Design review of the part built by this model. Coordinates are the model's own, in mm. Give positions to 0.01 mm unless a question says otherwise; leave off trailing zeros. Loops run counter-clockwise (first coordinate to the right, second up) from the corner with the lowest first, then second, coordinate; pieces in that order, holes last. Notation, with made-up numbers: M 31,-6.5 L 59,-6.5 A24 cw 59,31.5 Z; hole C -32.5,85.25 d4. An arc over 180 degrees is marked long. Use CSV: the item, a comma, the result in double quotes.
from build123d import *

# Parameters (mm, degrees)
SKETCH1_R           = 2.4892
SKETCH1_R_2         = 2.5527
BOSS_EXTRUDE1_DEPTH = 3.175
SKETCH2_W           = 4.445
SKETCH2_H           = 39.37
CUT_EXTRUDE1_DEPTH  = 4.175
FILLET2_R           = 4.7625


with BuildPart() as part:
    # Sketch1 → Boss-Extrude1 (new body)
    with BuildSketch(Plane.XY):
        Polygon((-34.925, 31.75), (-34.925, -29.21), (34.925, -29.21), (34.925, -7.62), (-10.795, -7.62), (-10.795, 31.75), align=None)
        with Locations((-25.4, -19.05)):
            Circle(SKETCH1_R, mode=Mode.SUBTRACT)
        with Locations((-7.874, -19.05)):
            Circle(SKETCH1_R, mode=Mode.SUBTRACT)
        with Locations((-25.4, -6.35)):
            Circle(SKETCH1_R, mode=Mode.SUBTRACT)
        with Locations((4.826, -19.05)):
            Circle(SKETCH1_R_2, mode=Mode.SUBTRACT)
        with Locations((17.526, -19.05)):
            Circle(SKETCH1_R_2, mode=Mode.SUBTRACT)
        with Locations((-25.4, 6.35)):
            Circle(SKETCH1_R, mode=Mode.SUBTRACT)
        with Locations((-25.4, 19.05)):
            Circle(SKETCH1_R, mode=Mode.SUBTRACT)
        with Locations((-25.4, -19.05)):
            Circle(SKETCH1_R)
    extrude(amount=BOSS_EXTRUDE1_DEPTH)

    # Sketch2 → Cut-Extrude1 (cut, through all)
    with BuildSketch(Plane.XY.offset(3.175)):
        with Locations((-13.0175, 12.065)):
            Rectangle(SKETCH2_W, SKETCH2_H)
    extrude(amount=-CUT_EXTRUDE1_DEPTH, mode=Mode.SUBTRACT)

    # Fillet2
    fillet2_edges = [part.edges().sort_by_distance(p)[0] for p in [
        (-34.925, 31.75, 1.5875),
        (34.925, -7.62, 1.5875),
        (34.925, -29.21, 1.5875),
        (-34.925, -29.21, 1.5875),
        (-15.24, -7.62, 1.5875),
        (-15.24, 31.75, 1.5875),
    ]]
    fillet(fillet2_edges, radius=FILLET2_R)


solid = part.part
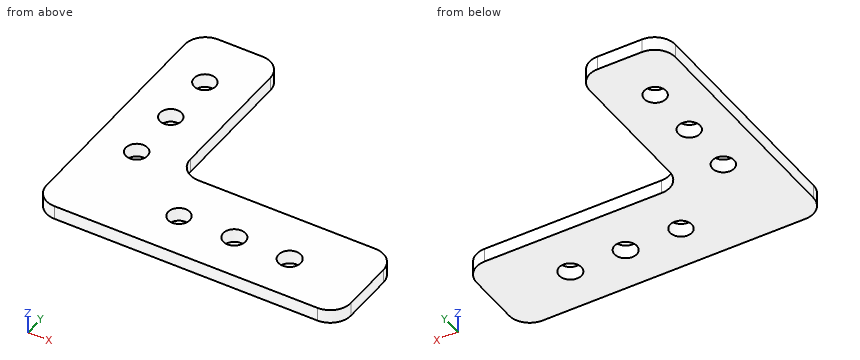
(1) We need section B-B on y = 19.05. State the section outline as (x, z) points (3 decimals), then the cut area to 3 significant figures.
A:
outline,"M -34.925,0 L -27.889,0 L -27.889,3.175 L -34.925,3.175 Z; M -22.911,0 L -15.24,0 L -15.24,3.175 L -22.911,3.175 Z"
area,"46.7 mm²"
(2) We need section C-C on z = 0.6. Count the separate pieces of the cut face and the enclosed holes in it, then the cut area to 3 significant figures.
A:
separate pieces,"1"
enclosed holes,"6"
area,"2,140 mm²"
(3) Clearance check with a flat-ended pin moving along its axis: P1, Ø6.5, axis at x = -25.4, y = 19.05, coming from the +Z side (3 decimals). State where the tip first meets the part, or that it passes through.
A:
P1,"z = 3.175"
(4) We need section D-D on x = 10.5. State the section outline as (y, z) points (3 decimals).
A:
outline,"M -29.21,0 L -7.62,0 L -7.62,3.175 L -29.21,3.175 Z"
(5) We need section A-A on y = -19.05. State the section outline as (x, z) points (3 decimals), then the cut area to 3 significant figures.
A:
outline,"M -34.925,0 L -10.363,0 L -10.363,3.175 L -34.925,3.175 Z; M -5.385,0 L 2.273,0 L 2.273,3.175 L -5.385,3.175 Z; M 7.379,0 L 14.973,0 L 14.973,3.175 L 7.379,3.175 Z; M 20.079,0 L 34.925,0 L 34.925,3.175 L 20.079,3.175 Z"
area,"174 mm²"
(6) Wall thickness on line 1 along Y through (x, z) = (-25.4, 1.3); line 2 along Y through (x, z) = (20.5, 1.8); line 3 along Y through (x, z) = (17, 1.15): over which ranges is each line inside the solid? List them lowest first. Write a range as [from, to].
A:
line 1,"[-29.21, -8.84], [-3.86, 3.86], [8.84, 16.56], [21.54, 31.75]"
line 2,"[-29.21, -7.62]"
line 3,"[-29.21, -21.55], [-16.55, -7.62]"
